from build123d import *

# Parameters (mm, degrees)
SKETCH_W       = 160
SKETCH_H       = 75
PAD_DEPTH      = 5
SKETCH001_R    = 2.25
HOLE_DEPTH     = 5.001
SKETCH002_R    = 1.25
HOLE001_DEPTH  = 25
HOLE001_TIPS_R = 1.25


with BuildPart() as part:
    # Sketch → Pad (new body)
    with BuildSketch(Plane.XY):
        Rectangle(SKETCH_W, SKETCH_H)
    extrude(amount=PAD_DEPTH)

    # Sketch001 (on Face5 of Pad) → Hole (cut, through all)
    with BuildSketch(Plane(origin=(0, 0, 0), x_dir=(1, 0, 0), z_dir=(0, 0, -1))):
        with Locations((-75, 32.5)):
            Circle(SKETCH001_R)
        with Locations((75, 32.5)):
            Circle(SKETCH001_R)
        with Locations((75, -32.5)):
            Circle(SKETCH001_R)
        with Locations((-75, -32.5)):
            Circle(SKETCH001_R)
    extrude(amount=-HOLE_DEPTH, mode=Mode.SUBTRACT)

    # Sketch002 (on Face1 of Hole) → Hole001 (cut)
    with BuildSketch(Plane(origin=(0, 37.5, 0), x_dir=(-1, 0, 0), z_dir=(0, 1, 0))):
        with Locations((-47.5, 2.5)):
            Circle(SKETCH002_R)
        with Locations((47.5, 2.5)):
            Circle(SKETCH002_R)
    extrude(amount=-HOLE001_DEPTH, mode=Mode.SUBTRACT)

    # Hole001 tips → Hole001 tip 1 section 0
    with BuildSketch(Plane(origin=(0, 12.5, 0), x_dir=(-1, 0, 0), z_dir=(0, 1, 0)), mode=Mode.PRIVATE) as hole001_tip_1_s0:
        with Locations((-47.5, 2.5)):
            Circle(HOLE001_TIPS_R)
    loft([hole001_tip_1_s0.sketch, Vertex(47.5, 11.748924, 2.5)], mode=Mode.SUBTRACT)

    # Hole001 tips → Hole001 tip 2 section 0
    with BuildSketch(Plane(origin=(0, 12.5, 0), x_dir=(-1, 0, 0), z_dir=(0, 1, 0)), mode=Mode.PRIVATE) as hole001_tip_2_s0:
        with Locations((47.5, 2.5)):
            Circle(HOLE001_TIPS_R)
    loft([hole001_tip_2_s0.sketch, Vertex(-47.5, 11.748924, 2.5)], mode=Mode.SUBTRACT)


solid = part.part
The listing builds one solid part. Answer for the finished solid, in the listing's coordinates (mm). Round coordinates to 2 decimals unless told otherwise and drop trailing zeros. Order: outer loops, then holes, each group sorted by start corner. A loop starts at its lowest first (then second) coordinate and runs counter-clockwise, first axis right, second up. Notation, with made-up numbers: M 28,46 L 53,46 A31 cw 53,82 Z; hole C 57.25,11 d10. An arc over 180 degrees is marked long. Answer in a Markdown table with one row per item. Add a question column.
1) The part is cut by section A-A on x = 75. Determine the outline of the cut face in (y, z).
2) Determine the mould class of faces 1 (the face through (-1, 37.5, 2)), 2 (the face through (-1, -37.5, 2)), 3 (the face through (-1, 1, 0)), 4 (the face through (76.21, 30.603, 2.465)) for opening direction Y: pulls with the +Y half, pulls with the -Y half, needs draft (parallel to the pull), parting line crosses it, or undercut.
3) A flat-ended cylindrical pin translates along its axis: pin 1 Ø4 at (x, y) = (-75, 32.5) entering from -Z. Find the tip coordinate at first contact, or state that the pin passes through.
4) The part is cut by section B-B on y = 32.5. Determine the outline of the cut face in (x, z).
5) Consider line 1 along Y through (x, z) = (75, 3.6); line 2 along X through (y, z) = (-32.5, 2.6); line 3 along X through (y, z) = (23.5, 2.25). Determine where each line is inside the solid, lowest interval first. Write a range as from..to.
Findings below:
| question | item | result |
|---|---|---|
| 1 | outline | M -37.5,0 L -34.75,0 L -34.75,5 L -37.5,5 Z; M -30.25,0 L 30.25,0 L 30.25,5 L -30.25,5 Z; M 34.75,0 L 37.5,0 L 37.5,5 L 34.75,5 Z |
| 2 | face 1 | pulls with the +Y half |
| 2 | face 2 | pulls with the -Y half |
| 2 | face 3 | needs draft |
| 2 | face 4 | undercut |
| 3 | pin 1 | passes through |
| 4 | outline | M -80,0 L -77.25,0 L -77.25,5 L -80,5 Z; M -72.75,0 L 72.75,0 L 72.75,5 L -72.75,5 Z; M 77.25,0 L 80,0 L 80,5 L 77.25,5 Z; hole C -47.5,2.5 d2.5; hole C 47.5,2.5 d2.5 |
| 5 | line 1 | y = -37.5..-34.75, -30.25..30.25, 34.75..37.5 |
| 5 | line 2 | x = -80..-77.25, -72.75..72.75, 77.25..80 |
| 5 | line 3 | x = -80..-48.72, -46.28..46.28, 48.72..80 |
